Verification items for the finished model (mm, model axes). Face numbers are marked on the shaded views. A direction names the side the tool comes from. Give positions to 0.01 mm unless a question says otherwise; leave off trailing zeros. Loops run counter-clockwise (first coordinate to the right, second up) from the corner with the lowest first, then second, coordinate; pieces in that order, holes last. Notation, with made-up numbers: (87, -37.5) -> (125, -37.5) arc R28 cw to (125, -19.5) -> close; hole circle Ø9 at (68.25, -6.5). An arc over 180 degrees is marked (long way). Answer in a Markdown table with one row per item. Add a question column.
Q1. Section check C-C on z = -1.25. Enter the section's corners in (x, y) (3 decimals), and give its area (3 significant figures).
Q2. Section check B-B on y = -8.5. Enter the section's corners in (x, z) (3 decimals).
Q3. Gauge pin test, flat ends, axial feed: P1, Ø0.6, axis at y = 15.5, z = 2.5, coming from the +X side; P2, Ø8, axis at x = -6, y = 10, coming from the +Z side; P3, Ø1.4, axis at x = -10, z = 3, coming from the +Y side (3 decimals); P4, Ø5, axis at x = 11.5, y = -12.5, coming from the +Z side. Record the tip position at first contact, or that the pin passes through.
Q4. Section check D-D on x = 6.5. Enter the section's corners in (y, z) (3 decimals), and give its area (3 significant figures).
Q5. Release check for a two-part mould opening along Y. For the marked faces 4, 5 and 6 record: pulls with the +Y half, pulls with the -Y half, needs draft (parallel to the pull), parting line crosses it, or undercut.
Q6. Section check A-A on x = 17.5. Enter the section's corners in (y, z) (3 decimals).
Q7. Material ranges on probe 1 along Y at (x, z) = (-17.5, 0.8) (3 decimals); probe 2 along Z at (x, y) = (-3.5, -23); probe 3 along Y at (x, z) = (-5, 5.75) (3 decimals), recorded low to high.
Q8. Set-up check for the marked faces 1, 2 and 3: record each of +Z, -Z, +X, -X, +Y, -Y from which the full face is reachable in a straight line by a thin tool's end or side.
```python
from build123d import *

# Parameters (mm, degrees)
F0_W      = 44.25
F0_H      = 38.75
F0_R      = 1.75
F1_DEPTH  = 1.75
F2_R      = 2
F3_W      = 14
F3_H      = 9
F4_DEPTH  = 6
F3_W_2    = 7
F3_H_2    = 8
F5_DEPTH  = 5
F3_W_3    = 1.75
F3_H_3    = 3
F6_DEPTH  = 2
F3_W_4    = 11
F3_H_4    = 6
F3_H_5    = 4
F7_DEPTH  = 5
F8_R      = 3
F9_DEPTH  = 9.4
F8_R_2    = 2.25
F10_DEPTH = 12
F8_W      = 15.25
F8_H      = 21
F8_H_2    = 10
F11_DEPTH = 3.7
F12_R     = 2
F13_R     = 2


with BuildPart() as f1:
    # F0 (on Top) → F1 (new body)
    with BuildSketch(Plane.XY):
        Rectangle(F0_W, F0_H)
        with Locations((-17.5, -14)):
            Circle(F0_R, mode=Mode.SUBTRACT)
        with Locations((17.5, -14)):
            Circle(F0_R, mode=Mode.SUBTRACT)
        with Locations((-17.5, 14)):
            Circle(F0_R, mode=Mode.SUBTRACT)
        with Locations((17.5, 14)):
            Circle(F0_R, mode=Mode.SUBTRACT)
    extrude(amount=F1_DEPTH)

    # F2
    f2_edges = [f1.edges().sort_by_distance(p)[0] for p in [
        (22.125, -19.375, 0.875),
        (-22.125, -19.375, 0.875),
        (-22.125, 19.375, 0.875),
        (22.125, 19.375, 0.875),
    ]]
    fillet(f2_edges, radius=F2_R)

    # F3 (on face) → F4 (join)
    with BuildSketch(Plane.XY.offset(1.75)):
        with Locations((6.9, 14.375)):
            Rectangle(F3_W, F3_H)
        with Locations((9.625, -6.47)):
            Rectangle(F3_W, F3_H)
    extrude(amount=F4_DEPTH)

    # F3 (on face) → F5 (join)
    with BuildSketch(Plane.XY.offset(1.75)):
        with Locations((-18.125, 5.25)):
            Rectangle(F3_W_2, F3_H_2)
        with Locations((18.125, 5.25)):
            Rectangle(F3_W_2, F3_H_2)
    extrude(amount=F5_DEPTH)

    # F3 (on face) → F6 (join)
    with BuildSketch(Plane.XY.offset(1.75)):
        with Locations((-10.125, 15.475)):
            Rectangle(F3_W_3, F3_H_3)
    extrude(amount=F6_DEPTH)

    # F3 (on face) → F7 (join)
    with BuildSketch(Plane.XY.offset(1.75)):
        with Locations((-6.625, -16.375)):
            Rectangle(F3_W_4, F3_H_4)
        with Locations((-6.625, -21.375)):
            Rectangle(F3_W_4, F3_H_5)
    extrude(amount=F7_DEPTH)

    # F8 (on face) → F9 (join)
    with BuildSketch(Plane(origin=(0, 0, 0), x_dir=(1, 0, 0), z_dir=(0, 0, -1))):
        with Locations((-1.553635, -5.567789)):
            Circle(F8_R)
        with Locations((12.125, 15.375)):
            Circle(F8_R)
    extrude(amount=F9_DEPTH)

    # F8 (on face) → F10 (join)
    with BuildSketch(Plane(origin=(0, 0, 0), x_dir=(1, 0, 0), z_dir=(0, 0, -1))):
        with Locations((-8.803919, -12.125)):
            Circle(F8_R_2)
    extrude(amount=F10_DEPTH)

    # F8 (on face) → F11 (join)
    with BuildSketch(Plane(origin=(0, 0, 0), x_dir=(1, 0, 0), z_dir=(0, 0, -1))):
        with Locations((-7.5, 8.875)):
            Rectangle(F8_W, F8_H)
        with Locations((-7.5, 24.375)):
            Rectangle(F8_W, F8_H_2)
    extrude(amount=F11_DEPTH)

    # F12
    f12_edges = [f1.edges().sort_by_distance(p)[0] for p in [
        (9.125, -15.375, -9.4),
        (-4.553635, 5.567789, -9.4),
    ]]
    fillet(f12_edges, radius=F12_R)

    # F13
    f13_edges = [f1.edges().sort_by_distance(p)[0] for p in [
        (-11.053919, 12.125, -12),
    ]]
    fillet(f13_edges, radius=F13_R)


solid = f1.part
```
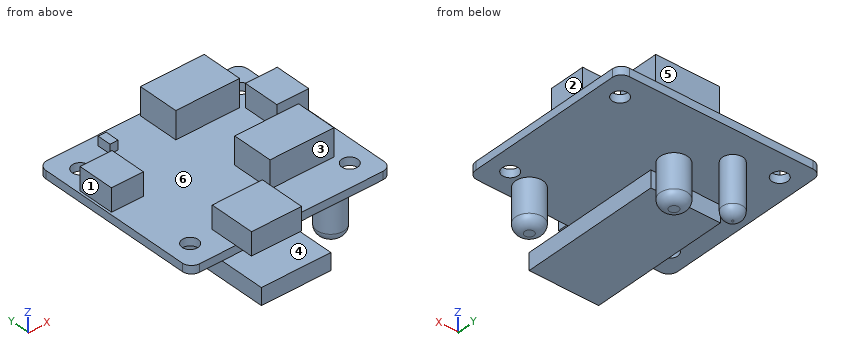
Taken from the geometry:
| question | item | result |
|---|---|---|
| 1 | outline | (-15.125, -29.375) -> (0.125, -29.375) -> (0.125, 1.625) -> (-15.125, 1.625) -> close; circle Ø4.5 at (-8.804, 12.125); circle Ø6 at (-1.554, 5.568); circle Ø6 at (12.125, -15.375) |
| 1 | area | 545 mm² |
| 2 | outline | (-22.125, 0) -> (-15.125, 0) -> (-15.125, -3.7) -> (0.125, -3.7) -> (0.125, 0) -> (22.125, 0) -> (22.125, 1.75) -> (16.625, 1.75) -> (16.625, 7.75) -> (2.625, 7.75) -> (2.625, 1.75) -> (-22.125, 1.75) -> close |
| 3 | P1 | stops at x = 13.9 |
| 3 | P2 | stops at z = 1.75 |
| 3 | P3 | stops at y = 16.975 |
| 3 | P4 | stops at z = 7.75 |
| 4 | outline | (-19.375, 0) -> (19.375, 0) -> (19.375, 1.75) -> (18.875, 1.75) -> (18.875, 7.75) -> (9.875, 7.75) -> (9.875, 1.75) -> (-1.97, 1.75) -> (-1.97, 7.75) -> (-10.97, 7.75) -> (-10.97, 1.75) -> (-19.375, 1.75) -> close |
| 4 | area | 176 mm² |
| 5 | face 4 | needs draft |
| 5 | face 5 | pulls with the +Y half |
| 5 | face 6 | undercut |
| 6 | outline | (-19.375, 0) -> (-15.75, 0) -> (-15.75, 1.75) -> (-19.375, 1.75) -> close; (-12.25, 0) -> (12.25, 0) -> (12.25, 1.75) -> (9.25, 1.75) -> (9.25, 6.75) -> (1.25, 6.75) -> (1.25, 1.75) -> (-12.25, 1.75) -> close; (15.75, 0) -> (19.375, 0) -> (19.375, 1.75) -> (15.75, 1.75) -> close |
| 7 | probe 1 | y = -19.375 to -15.75, -12.25 to 12.25, 15.75 to 19.375 |
| 7 | probe 2 | z = -3.7 to 0, 1.75 to 6.75 |
| 7 | probe 3 | y = -23.375 to -13.375 |
| 8 | face 1 | +Z, -X, +Y, -Y |
| 8 | face 2 | +Z, +X, +Y, -Y |
| 8 | face 3 | +Z, +X, -X, -Y |
